Could you check a few things on this model? Use its own coordinates, in mm. A direction names the side the tool comes from. Give positions to 0.01 mm unless a question says otherwise; leave off trailing zeros. Order: outer loops, then holes, each group sorted by start corner. A loop starts at its lowest first (then second) coordinate and runs counter-clockwise, first axis right, second up. Notation, with made-up numbers: (1.25, 13) -> (35.25, 13) arc R14 cw to (35.25, 17) -> close; hole circle Ø2 at (-28.5, 61.5). An arc over 180 degrees is marked (long way). Write each question's results on one line, items separated by ' | '.
```python
from build123d import *

# Parameters (mm, degrees)
F0_W     = 85.09
F0_H     = 56.134
F1_DEPTH = 1.5875
F2_W     = 73.66
F2_H     = 41.91
F3_DEPTH = 6.35
F4_R     = 2.921
F4_R_2   = 1.016
F5_DEPTH = 3.175
F6_DEPTH = 6.35


with BuildPart() as f1:
    # F0 (on Top) → F1 (new body)
    with BuildSketch(Plane.XY):
        Rectangle(F0_W, F0_H)
    extrude(amount=F1_DEPTH)

    # F2 (on face) → F3 (cut)
    with BuildSketch(Plane.XY.offset(1.5875)):
        Rectangle(F2_W, F2_H)
    extrude(amount=-F3_DEPTH, mode=Mode.SUBTRACT)

    # F4 (on face) → F5 (join)
    with BuildSketch(Plane.XY.offset(1.5875)):
        with Locations((38.989, 24.511)):
            Circle(F4_R)
        with Locations((38.989, 24.511)):
            Circle(F4_R_2, mode=Mode.SUBTRACT)
        with Locations((38.989, -24.511)):
            Circle(F4_R)
        with Locations((38.989, -24.511)):
            Circle(F4_R_2, mode=Mode.SUBTRACT)
        with Locations((-19.177, 24.511)):
            Circle(F4_R)
        with Locations((-19.177, 24.511)):
            Circle(F4_R_2, mode=Mode.SUBTRACT)
        with Locations((-19.177, -24.511)):
            Circle(F4_R)
        with Locations((-19.177, -24.511)):
            Circle(F4_R_2, mode=Mode.SUBTRACT)
    extrude(amount=F5_DEPTH)

    # F4 (on face) → F6 (cut)
    with BuildSketch(Plane.XY.offset(1.5875)):
        with Locations((38.989, -24.511)):
            Circle(F4_R_2)
        with Locations((-19.177, 24.511)):
            Circle(F4_R_2)
        with Locations((38.989, 24.511)):
            Circle(F4_R_2)
        with Locations((-19.177, -24.511)):
            Circle(F4_R_2)
    extrude(amount=-F6_DEPTH, mode=Mode.SUBTRACT)


solid = f1.part
```
Q1. Suppose I cut it at A-A on x = -26. Please give me the cut outline in (y, z) (1 decimal), and give its area (3 significant figures).
Here are the results:
outline: (-28.1, 0) -> (-21, 0) -> (-21, 1.6) -> (-28.1, 1.6) -> close; (21, 0) -> (28.1, 0) -> (28.1, 1.6) -> (21, 1.6) -> close | area: 22.6 mm²
Q2. Thinking about a two-plate mould opening in X: for faces 1 (the flat face through (-19, 23, 4.762)), 2 (the cylindrical face through (38.609, -21.615, 3.153)), 3 (the flat face through (42.545, 0, 1)), which applies, +X half, -X half, draft (parallel to the pull), parting line (faces both ways), or undercut?
Here are the results:
face 1: draft | face 2: undercut | face 3: +X half
Q3. Suppose I cut it at B-B on z = 3.8. Please give me the cut outline in (x, y) (3 decimals), and give its area (3 significant figures).
Here are the results:
outline: circle Ø5.842 at (-19.177, -24.511); circle Ø5.842 at (-19.177, 24.511); circle Ø5.842 at (38.989, -24.511); circle Ø5.842 at (38.989, 24.511); hole circle Ø2.032 at (-19.177, -24.511); hole circle Ø2.032 at (-19.177, 24.511); hole circle Ø2.032 at (38.989, -24.511); hole circle Ø2.032 at (38.989, 24.511) | area: 94.2 mm²
Q4. I'm going to push a flat-ended pin straight in: pin 1 Ø4 at (x, y) = (9.5, 20) entering from +Z. Where does the tip first touch, or does it pass through?
Here are the results:
pin 1: stops at z = 1.59
Q5. Suppose I cut it at C-C on y = 6.5. Please give me the cut outline in (x, z) (1 decimal).
Here are the results:
outline: (-42.5, 0) -> (-36.8, 0) -> (-36.8, 1.6) -> (-42.5, 1.6) -> close; (36.8, 0) -> (42.5, 0) -> (42.5, 1.6) -> (36.8, 1.6) -> close
Q6. I need wall thicknesses on line 1 along Y through (x, z) = (39.5, 2.8); line 2 along X through (y, z) = (8, 1.4) (3 decimals); line 3 along Y through (x, z) = (-12.5, 1) (3 decimals). Which ranges of each line are inside material? Lowest first, please.
Here are the results:
line 1: y = -27.39 to -25.39, -23.63 to -21.64, 21.64 to 23.63, 25.39 to 27.39 | line 2: x = -42.545 to -36.83, 36.83 to 42.545 | line 3: y = -28.067 to -20.955, 20.955 to 28.067
Q7. For faces 4 (the flat face through (-19, -26, 4.762)), 5 (the cylindrical face through (-19.557, -21.615, 3.153)), 6 (the flat face through (36.83, 0, 1)), which set-ups out of +Z, -Z, +X, -X, +Y, -Y let a thin tool reach every point of the face, with its end or its side?
Here are the results:
face 4: +Z, +X, -X, +Y, -Y | face 5: +Z | face 6: +Z, -Z
